Source: CAD feature listing. Evaluate the final solid. Frame: model axes, mm. Coordinates: 2 decimals unless noted, no trailing zeros. Order: outer loops, then holes, each group sorted by start corner. A loop starts at its lowest first (then second) coordinate and runs counter-clockwise, first axis right, second up. Notation, with made-up numbers: (22, -38.5) -> (27, -38.5) arc R30 ccw to (27, -12.5) -> close; hole circle Ø1 at (58.25, 84.25). An arc over 180 degrees is marked (long way). Write item = value, one per line. Start each with the question number.
Item 1: Contact query for flat-ended pins moving along their axis: pin 1 (1.5 mm diameter, centred on y = 63, z = 2.5, fed in from -X); pin 2 (1 mm diameter, centred on y = 137, z = 2.5, fed in from +X). Output: stop coordinate, or through.
Item 2: Section query A-A (z = 2). Count the separate pieces of the cut face and the enclosed holes in it, then the cut area to 3 significant figures.
Item 3: Ray query, line 1 along X through (y, z) = (220.5, 1); line 2 along X through (y, z) = (63, 2.15); line 3 along Y through (x, z) = (13.5, 1.8). Return the intervals inside material, ascending. Write a range as [from, to].
Item 4: Section query B-B (y = 150). Output: boundary loops of the cut face in (x, z).
```python
from build123d import *

# Parameters (mm, degrees)
SKETCH2_W           = 3
SKETCH2_H           = 3
BOSS_EXTRUDE2_DEPTH = 3


with BuildPart() as part:
    # Sketch2 → Boss-Extrude2 (new body)
    with BuildSketch(Plane.XY):
        Polygon((10, 250), (15, 250), (15, 253), (25, 253), (28, 253), (28, 235), (25, 235), (25, 215), (28, 215), (28, 195), (25, 195), (25, 175), (28, 175), (28, 155), (25, 155), (25, 135), (28, 135), (28, 115), (25, 115), (25, 95), (28, 95), (28, 75), (25, 75), (25, 55), (28, 55), (28, 35), (25, 35), (25, 15), (28, 15), (28, -3), (25, -3), (15, -3), (15, 0), (10, 0), (10, -3), (0, -3), (-3, -3), (-3, 15), (0, 15), (0, 35), (-3, 35), (-3, 55), (0, 55), (0, 75), (-3, 75), (-3, 95), (0, 95), (0, 115), (-3, 115), (-3, 135), (0, 135), (0, 155), (-3, 155), (-3, 175), (0, 175), (0, 195), (-3, 195), (-3, 215), (0, 215), (0, 235), (-3, 235), (-3, 253), (0, 253), (10, 253), align=None)
        with Locations((20.5, 191.5)):
            Rectangle(SKETCH2_W, SKETCH2_H, mode=Mode.SUBTRACT)
        with Locations((20.5, 221.5)):
            Rectangle(SKETCH2_W, SKETCH2_H, mode=Mode.SUBTRACT)
        with Locations((20.5, 161.5)):
            Rectangle(SKETCH2_W, SKETCH2_H, mode=Mode.SUBTRACT)
        with Locations((20.5, 131.5)):
            Rectangle(SKETCH2_W, SKETCH2_H, mode=Mode.SUBTRACT)
        with Locations((20.5, 101.5)):
            Rectangle(SKETCH2_W, SKETCH2_H, mode=Mode.SUBTRACT)
        with Locations((20.5, 71.5)):
            Rectangle(SKETCH2_W, SKETCH2_H, mode=Mode.SUBTRACT)
        with Locations((20.5, 41.5)):
            Rectangle(SKETCH2_W, SKETCH2_H, mode=Mode.SUBTRACT)
        with Locations((20.5, 11.5)):
            Rectangle(SKETCH2_W, SKETCH2_H, mode=Mode.SUBTRACT)
    extrude(amount=BOSS_EXTRUDE2_DEPTH)


solid = part.part
```
Computed:
q1.pin_1 = 0
q1.pin_2 = 25
q2.separate_pieces = 1
q2.enclosed_holes = 8
q2.area = 7,110 mm^2
q3.line_1 = [0, 19], [22, 25]
q3.line_2 = [0, 25]
q3.line_3 = [0, 250]
q4.outline = (0, 0) -> (25, 0) -> (25, 3) -> (0, 3) -> close
